```python
from build123d import *

# Parameters (mm, degrees)
EXTRUDE_1_DEPTH      = 4
SKETCH_6_R           = 1.75
CUT_EXTRUDE_3_DEPTH  = 4
SKETCH_4_R           = 1.75
CUT_EXTRUDE_4_DEPTH  = 4
SKETCH_7_R           = 1.75
CUT_EXTRUDE_5_DEPTH  = 4
SKETCH_8_R           = 1.75
CUT_EXTRUDE_6_DEPTH  = 4
CUT_EXTRUDE_7_DEPTH  = 4
SKETCH_10_R          = 1.75
SKETCH_10_R_2        = 1.749999998
CUT_EXTRUDE_9_DEPTH  = 4
SKETCH_11_W          = 20.115281517
SKETCH_11_H          = 10.033042315
SKETCH_11_R          = 1.75
CUT_EXTRUDE_10_DEPTH = 2
SKETCH_11_5_R        = 1.75
CUT_EXTRUDE_11_DEPTH = 10
SKETCH_12_R          = 1.75
CUT_EXTRUDE_13_DEPTH = 379.008231755


with BuildPart() as part:
    # Sketch 3 → Extrude 1 (new body)
    with BuildSketch(Plane.XY):
        with BuildLine():
            Line((73.505746565, 259.089488009), (196.937204075, 259.089488009))
            ThreePointArc((196.937204075, 259.089488009), (204.590872722, 257.56707866), (211.079339699, 253.231623633))
            Line((211.079339699, 253.231623633), (269.363610944, 194.947352388))
            ThreePointArc((269.363610944, 194.947352388), (273.69906597, 188.458885412), (275.22147532, 180.805216764))
            Line((275.22147532, 180.805216764), (275.22147532, 54.089488009))
            ThreePointArc((275.22147532, 54.089488009), (269.363610944, 39.947352386), (255.22147532, 34.089488009))
            Line((255.22147532, 34.089488009), (15.221475318, 34.089488009))
            ThreePointArc((15.221475318, 34.089488009), (1.079339694, 39.947352386), (-4.778524682, 54.089488009))
            Line((-4.778524682, 54.089488009), (-4.778524682, 180.805216762))
            ThreePointArc((-4.778524682, 180.805216762), (-3.256115333, 188.458885409), (1.079339694, 194.947352386))
            Line((1.079339694, 194.947352386), (59.363610941, 253.231623633))
            ThreePointArc((59.363610941, 253.231623633), (65.852077918, 257.56707866), (73.505746565, 259.089488009))
        make_face()
    extrude(amount=EXTRUDE_1_DEPTH)

    # Sketch 6 → Cut-Extrude 3 (cut)
    with BuildSketch(Plane.XY.offset(4)):
        with Locations((223.22147532, 174.880072532)):
            Circle(SKETCH_6_R)
        with Locations((260.22147532, 174.880072532)):
            Circle(SKETCH_6_R)
        with Locations((260.22147532, 113.880072532)):
            Circle(SKETCH_6_R)
        with Locations((223.22147532, 113.880072532)):
            Circle(SKETCH_6_R)
    extrude(amount=-CUT_EXTRUDE_3_DEPTH, mode=Mode.SUBTRACT)

    # Sketch 4 → Cut-Extrude 4 (cut)
    with BuildSketch(Plane.XY.offset(4)):
        with Locations((174.691475319, 240.74535793)):
            Circle(SKETCH_4_R)
        with Locations(Location((174.691475319, 188.63535793, 0), (0, 0, 180))):
            Circle(SKETCH_4_R)
        with Locations((95.751475319, 188.63535793)):
            Circle(SKETCH_4_R)
        with Locations(Location((95.751475319, 240.74535793, 0), (0, 0, 180))):
            Circle(SKETCH_4_R)
        with Locations((165.22147532, 53.06830954)):
            Circle(SKETCH_4_R)
        with Locations(Location((105.22147532, 53.06830954, 0), (0, 0, 180))):
            Circle(SKETCH_4_R)
    extrude(amount=-CUT_EXTRUDE_4_DEPTH, mode=Mode.SUBTRACT)

    # Sketch 7 → Cut-Extrude 5 (cut)
    with BuildSketch(Plane.XY.offset(4)):
        with Locations((122.221475319, 129.089488009)):
            Circle(SKETCH_7_R)
        with Locations((148.221475319, 129.089488009)):
            Circle(SKETCH_7_R)
        with Locations((122.221475319, 69.089488009)):
            Circle(SKETCH_7_R)
        with Locations((148.221475319, 69.089488009)):
            Circle(SKETCH_7_R)
    extrude(amount=-CUT_EXTRUDE_5_DEPTH, mode=Mode.SUBTRACT)

    # Sketch 8 → Cut-Extrude 6 (cut)
    with BuildSketch(Plane.XY.offset(4)):
        with Locations((22.867250591, 95.494716411)):
            Circle(SKETCH_8_R)
        with Locations((65.293657462, 53.06830954)):
            Circle(SKETCH_8_R)
        with Locations((247.720064334, 95.494716411)):
            Circle(SKETCH_8_R)
        with Locations((205.293657462, 53.06830954)):
            Circle(SKETCH_8_R)
    extrude(amount=-CUT_EXTRUDE_6_DEPTH, mode=Mode.SUBTRACT)

    # Sketch 9 → Cut-Extrude 7 (cut)
    with BuildSketch(Plane.XY.offset(4)):
        with BuildLine():
            Line((135.22147532, 176.324698125), (85.22147532, 176.324698125))
            ThreePointArc((85.22147532, 176.324698125), (78.150407508, 173.395765937), (75.22147532, 166.324698125))
            Line((75.22147532, 166.324698125), (75.22147532, 156.324698125))
            ThreePointArc((75.22147532, 156.324698125), (78.150407508, 149.253630313), (85.22147532, 146.324698125))
            Line((85.22147532, 146.324698125), (185.22147532, 146.324698125))
            ThreePointArc((185.22147532, 146.324698125), (192.292543132, 149.253630313), (195.22147532, 156.324698125))
            Line((195.22147532, 156.324698125), (195.22147532, 166.324698125))
            ThreePointArc((195.22147532, 166.324698125), (192.292543132, 173.395765937), (185.22147532, 176.324698125))
            Line((185.22147532, 176.324698125), (135.22147532, 176.324698125))
        make_face()
    extrude(amount=-CUT_EXTRUDE_7_DEPTH, mode=Mode.SUBTRACT)

    # Sketch 10 → Cut-Extrude 9 (cut)
    with BuildSketch(Plane.XY.offset(4)):
        with Locations((106.721475319, 79.089488009)):
            Circle(SKETCH_10_R)
        with Locations((163.721475321, 79.089488009)):
            Circle(SKETCH_10_R_2)
        with Locations((106.721475319, 119.089488009)):
            Circle(SKETCH_10_R)
        with Locations(Location((163.721475321, 119.089488009, 0), (0, 0, 180))):
            Circle(SKETCH_10_R)
    extrude(amount=-CUT_EXTRUDE_9_DEPTH, mode=Mode.SUBTRACT)

    # Sketch 11 → Cut-Extrude 10 (cut)
    # profile 1 of 4: a face of its own
    with BuildSketch(Plane.XY.offset(4)):
        with Locations((65.852077918, 188.458885409)):
            Rectangle(SKETCH_11_W, SKETCH_11_H)
        with Locations((70.852077918, 188.458885409)):
            Circle(SKETCH_11_R, mode=Mode.SUBTRACT)
    # profile 2 of 4: a face of its own
    with BuildSketch(Plane.XY.offset(4)):
        with Locations((65.852077918, 80.084611013)):
            Rectangle(SKETCH_11_W, SKETCH_11_H)
        with Locations((70.852077918, 80.084611013)):
            Circle(SKETCH_11_R, mode=Mode.SUBTRACT)
    # profile 3 of 4: a face of its own
    with BuildSketch(Plane.XY.offset(4)):
        with Locations((204.590872723, 80.084611013)):
            Rectangle(SKETCH_11_W, SKETCH_11_H)
        with Locations((199.590872722, 80.084611013)):
            Circle(SKETCH_11_R, mode=Mode.SUBTRACT)
    # profile 4 of 4: a face of its own
    with BuildSketch(Plane.XY.offset(4)):
        with Locations((204.590872723, 188.458885409)):
            Rectangle(SKETCH_11_W, SKETCH_11_H)
        with Locations((199.590872722, 188.458885409)):
            Circle(SKETCH_11_R, mode=Mode.SUBTRACT)
    extrude(amount=-CUT_EXTRUDE_10_DEPTH, mode=Mode.SUBTRACT)

    # Sketch 11_5 → Cut-Extrude 11 (cut)
    with BuildSketch(Plane.XY.offset(4)):
        with Locations((70.852077918, 188.458885409)):
            Circle(SKETCH_11_5_R)
        with Locations((70.852077918, 80.084611013)):
            Circle(SKETCH_11_5_R)
        with Locations((199.590872722, 80.084611013)):
            Circle(SKETCH_11_5_R)
        with Locations((199.590872722, 188.458885409)):
            Circle(SKETCH_11_5_R)
    extrude(amount=-CUT_EXTRUDE_11_DEPTH, mode=Mode.SUBTRACT)

    # Sketch 12 → Cut-Extrude 13 (cut, through all)
    with BuildSketch(Plane.XY.offset(4)):
        with Locations((60.961423691, 169.312171827)):
            Circle(SKETCH_12_R)
        with Locations((60.961423691, 123.312171827)):
            Circle(SKETCH_12_R)
        with Locations((14.961423691, 123.312171827)):
            Circle(SKETCH_12_R)
        with Locations((14.961423691, 169.312171827)):
            Circle(SKETCH_12_R)
    extrude(amount=-CUT_EXTRUDE_13_DEPTH, mode=Mode.SUBTRACT)


solid = part.part
```
Model file for the job. Use its own axes, mm. A direction names the side the tool comes from. Coordinates: 2 decimals unless noted, no trailing zeros. Order: outer loops, then holes, each group sorted by start corner. A loop starts at its lowest first (then second) coordinate and runs counter-clockwise, first axis right, second up. Notation, with made-up numbers: (58.25, 20) -> (94.25, 20) arc R25 cw to (94.25, 57) -> close; hole circle Ø5 at (27.25, -15.75). An arc over 180 degrees is marked (long way). Return JSON: item names as keys, results as strings.
Item 1: Pin check, flat tips, straight feed: P1, Ø8, axis at x = 64, y = 188.5, coming from the +Z side; P2, Ø3, axis at x = 106.72, y = 119.09, coming from the +Z side; P3, Ø1, axis at y = 190, z = 2.5, coming from the -X side; P4, Ø1.6, axis at x = 205.5, z = 2.5, coming from the +Y side. Stop position of each tip, or through.
Model answer:
{"P1": "stops at z = 2", "P2": "passes through", "P3": "stops at x = -2.79", "P4": "stops at y = 257.52"}
Item 2: Slice it at B-B (z = 3.4). Count the separate pieces of the cut face and the enclosed holes in it, then the cut area to 3 significant figures.
Model answer:
{"separate pieces": "1", "enclosed holes": "31", "area": "53,300 mm²"}
Item 3: 3-axis set-ups, long thin cutter, end or side, ignore diameter. For faces 1 (the face through (-3.298, 188.357, 1.972)), 2 (the face through (66, 80, 2)), 3 (the face through (78.229, 173.473, 2.028)): which of +Z, -Z, +X, -X, +Y, -Y reach the whole face in a straight line?
Model answer:
{"face 1": "+Z, -Z, -X, +Y", "face 2": "+Z", "face 3": "+Z, -Z"}
Item 4: Mould opens along X. For faces 4 (the face through (204, 80, 2)), 5 (the face through (137, 123, 4)), 6 (the face through (273.657, 188.56, 1.972)), 7 (the face through (66, 189, 2)) say: pulls with the +X half, pulls with the -X half, needs draft (parallel to the pull), parting line crosses it, or undercut.
Model answer:
{"face 4": "undercut", "face 5": "needs draft", "face 6": "pulls with the +X half", "face 7": "undercut"}
Item 5: Slice it at D-D (x = 29.5). Write the cut outline in (y, z).
Model answer:
{"outline": "(34.09, 0) -> (223.37, 0) -> (223.37, 4) -> (34.09, 4) -> close"}
Item 6: Slice it at A-A (x = 142.5). Write the cut outline in (y, z), then the cut area to 3 significant figures.
Model answer:
{"outline": "(34.09, 0) -> (146.32, 0) -> (146.32, 4) -> (34.09, 4) -> close; (176.32, 0) -> (259.09, 0) -> (259.09, 4) -> (176.32, 4) -> close", "area": "780 mm²"}
Item 7: Wall check: line 1 along Y through (x, z) = (74, 3.2); line 2 along Y through (x, z) = (72, 2.85); line 3 along X through (y, z) = (95, 1.75). Give the ranges that are in metal, low to high. Write a range as from..to.
Model answer:
{"line 1": "y = 34.09..75.07, 85.1..183.44, 193.48..259.09", "line 2": "y = 34.09..75.07, 85.1..183.44, 193.48..259.03", "line 3": "x = -4.78..21.19, 24.55..246.04, 249.4..275.22"}
Item 8: Slice it at C-C (y = 205.5). Write the cut outline in (x, z).
Model answer:
{"outline": "(11.63, 0) -> (258.81, 0) -> (258.81, 4) -> (11.63, 4) -> close"}
